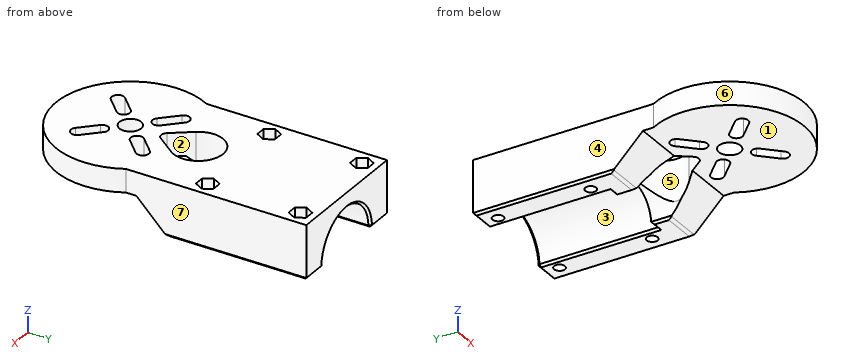
```python
from build123d import *

# Parameters (mm, degrees)
EXTRUDE006_DEPTH                     = 10
SKETCH006_AS_DRAWN_R                 = 9
EXTRUDE005_DEPTH                     = 27
EXTRUDE005_ONTO_SKETCH006_ROLL_ANGLE = 90
SKETCH_R                             = 3.5
SKETCH_R_2                           = 1.75
EXTRUDE_DEPTH                        = 30
SKETCH001_AS_DRAWN_R                 = 12.5
EXTRUDE004_DEPTH                     = 50
EXTRUDE004_ONTO_SKETCH001_ROLL_ANGLE = 90
EXTRUDE002_DEPTH                     = 60
SKETCH003_AS_DRAWN_W                 = 50
SKETCH003_AS_DRAWN_H                 = 17.5
EXTRUDE003_DEPTH                     = 98
EXTRUDE003_ONTO_SKETCH003_ROLL_ANGLE = 90
CHAMFER_SIZE                         = 0.7


with BuildPart() as extrude006:
    # Sketch008 → Extrude006 (new body)
    with BuildSketch(Plane(origin=(0, 40, 0), x_dir=(1, 0, 0), z_dir=(0, 0, 1))):
        Polygon((-17.625, -2.185417), (-14.375, -2.185417), (-12.75, -5), (-14.375, -7.814583), (-17.625, -7.814583), (-19.25, -5), align=None)
        Polygon((14.375, -2.185417), (17.625, -2.185417), (19.25, -5), (17.625, -7.814583), (14.375, -7.814583), (12.75, -5), align=None)
        Polygon((14.375, 27.814583), (17.625, 27.814583), (19.25, 25), (17.625, 22.185417), (14.375, 22.185417), (12.75, 25), align=None)
        Polygon((-17.625, 27.814583), (-14.375, 27.814583), (-12.75, 25), (-14.375, 22.185417), (-17.625, 22.185417), (-19.25, 25), align=None)
    extrude(amount=EXTRUDE006_DEPTH)


with BuildPart() as extrude006_1:
    # Extrude006 placement: moved
    add(extrude006.part.moved(Location((0, 0, 9))))


with BuildPart() as extrude005:
    # Sketch006 as drawn → Extrude005 (new)
    with BuildSketch(Plane.XY):
        Circle(SKETCH006_AS_DRAWN_R)
    extrude(amount=-EXTRUDE005_DEPTH)


with BuildPart() as extrude005_1:
    # Extrude005 onto Sketch006 roll: moved
    add(extrude005.part.rotate(Axis((0, 0, 0), (1, 0, 0)), EXTRUDE005_ONTO_SKETCH006_ROLL_ANGLE))


with BuildPart() as extrude005_2:
    # Extrude005 onto Sketch006 placement: moved
    add(extrude005_1.part.moved(Location((0, 33, 0))))


with BuildPart() as extrude005_3:
    # Extrude005 placement: moved
    add(extrude005_2.part.moved(Location((0, -18, 0))))


with BuildPart() as extrude_body:
    # Sketch → Extrude (new body)
    with BuildSketch(Plane.XY):
        Circle(SKETCH_R)
        with Locations((-16, 35)):
            Circle(SKETCH_R_2)
        with Locations((-16, 65)):
            Circle(SKETCH_R_2)
        with Locations((16, 65)):
            Circle(SKETCH_R_2)
        with Locations((16, 35)):
            Circle(SKETCH_R_2)
        with BuildLine():
            ThreePointArc((-12.020815, -9.192388), (-12.020815, -12.020815), (-9.192388, -12.020815))
            Line((-9.192388, -12.020815), (-4.242641, -7.071068))
            ThreePointArc((-4.242641, -7.071068), (-4.242641, -4.242641), (-7.071068, -4.242641))
            Line((-12.020815, -9.192388), (-7.071068, -4.242641))
        make_face()
        with BuildLine():
            ThreePointArc((7.071068, -4.242641), (4.242641, -4.242641), (4.242641, -7.071068))
            Line((4.242641, -7.071068), (9.192388, -12.020815))
            ThreePointArc((9.192388, -12.020815), (12.020815, -12.020815), (12.020815, -9.192388))
            Line((7.071068, -4.242641), (12.020815, -9.192388))
        make_face()
        with BuildLine():
            ThreePointArc((4.242641, 7.071068), (4.242641, 4.242641), (7.071068, 4.242641))
            Line((7.071068, 4.242641), (12.020815, 9.192388))
            ThreePointArc((12.020815, 9.192388), (12.020815, 12.020815), (9.192388, 12.020815))
            Line((4.242641, 7.071068), (9.192388, 12.020815))
        make_face()
        with BuildLine():
            ThreePointArc((-9.192388, 12.020815), (-12.020815, 12.020815), (-12.020815, 9.192388))
            Line((-12.020815, 9.192388), (-7.071068, 4.242641))
            ThreePointArc((-7.071068, 4.242641), (-4.242641, 4.242641), (-4.242641, 7.071068))
            Line((-9.192388, 12.020815), (-4.242641, 7.071068))
        make_face()
        with BuildLine():
            ThreePointArc((6.4, 17.2), (0, 30), (-6.4, 17.2))
            Line((-6.4, 17.2), (-1.6, 10.8))
            ThreePointArc((-1.6, 10.8), (0, 10), (1.6, 10.8))
            Line((6.4, 17.2), (1.6, 10.8))
        make_face()
        with BuildLine():
            ThreePointArc((-21, 11.61895), (0, -24), (21, 11.61895))
            Line((21, 70), (21, 11.61895))
            Line((30, 70), (21, 70))
            Line((30, -30), (30, 70))
            Line((-30, -30), (30, -30))
            Line((-30, 70), (-30, -30))
            Line((-21, 70), (-30, 70))
            Line((-21, 11.61895), (-21, 70))
        make_face()
    extrude(amount=EXTRUDE_DEPTH)


with BuildPart() as extrude004:
    # Sketch001 as drawn → Extrude004 (new)
    with BuildSketch(Plane.XY):
        Circle(SKETCH001_AS_DRAWN_R)
    extrude(amount=-EXTRUDE004_DEPTH)


with BuildPart() as extrude004_1:
    # Extrude004 onto Sketch001 roll: moved
    add(extrude004.part.rotate(Axis((0, 0, 0), (1, 0, 0)), EXTRUDE004_ONTO_SKETCH001_ROLL_ANGLE))


with BuildPart() as extrude004_2:
    # Extrude004 onto Sketch001 placement: moved
    add(extrude004_1.part.moved(Location((0, 32, 0))))


with BuildPart() as extrude004_3:
    # Extrude004 placement: moved
    add(extrude004_2.part.moved(Location((0, -1, 0))))


with BuildPart() as extrude002:
    # Sketch002 → Extrude002 (new body)
    with BuildSketch(Plane.YZ.offset(33)):
        Polygon((-30, 10), (15, 10), (25, 0), (-30, 0), align=None)
    extrude(amount=-EXTRUDE002_DEPTH)


with BuildPart() as chamfer_body:
    # Sketch003 as drawn → Extrude003 (new)
    with BuildSketch(Plane.XY):
        with Locations((0, 8.75)):
            Rectangle(SKETCH003_AS_DRAWN_W, SKETCH003_AS_DRAWN_H)
    extrude(amount=-EXTRUDE003_DEPTH)


with BuildPart() as chamfer_body_1:
    # Extrude003 onto Sketch003 roll: moved
    add(chamfer_body.part.rotate(Axis((0, 0, 0), (1, 0, 0)), EXTRUDE003_ONTO_SKETCH003_ROLL_ANGLE))


with BuildPart() as chamfer_body_2:
    # Extrude003 onto Sketch003 placement: moved
    add(chamfer_body_1.part.moved(Location((0, -28, 0))))

    # Cut: cut Extrude002
    add(extrude002.part, mode=Mode.SUBTRACT)

    # Cut001: cut Extrude004
    add(extrude004_3.part, mode=Mode.SUBTRACT)

    # Cut002: cut Extrude body
    add(extrude_body.part, mode=Mode.SUBTRACT)

    # Cut003: cut Extrude005
    add(extrude005_3.part, mode=Mode.SUBTRACT)

    # Cut004: cut Extrude006
    add(extrude006_1.part, mode=Mode.SUBTRACT)

    # Chamfer
    chamfer_edges = [chamfer_body_2.edges().sort_by_distance(p)[0] for p in [
        (-21, 47.5, 0),
        (16.75, 70, 0),
        (0, 70, 12.5),
        (-16.75, 70, 0),
        (21, 47.5, 0),
        (-15, 25, 0),
        (-9, 28, 0),
        (-12.5, 50.5, 0),
        (-10.75, 31, 0),
        (15, 25, 0),
        (9, 28, 0),
        (10.75, 31, 0),
        (12.5, 50.5, 0),
    ]]
    chamfer(chamfer_edges, length=CHAMFER_SIZE)


solid = chamfer_body_2.part
```
Read the model definition and answer for the solid it produces. Units are mm, in the model's axes. Face numbers are marked on the shaded views. A direction names the side the tool comes from. Coordinates: 2 decimals unless noted, no trailing zeros. Order: outer loops, then holes, each group sorted by start corner. A loop starts at its lowest first (then second) coordinate and runs counter-clockwise, first axis right, second up. Notation, with made-up numbers: (74.25, 42.5) - (113.25, 42.5) arc R23 cw to (113.25, 57.5) - close; hole circle Ø3 at (-22, -9.5). An arc over 180 degrees is marked (long way). Answer as a JSON object with one key per item and string values. Group by question number.
Item 1: Section A-A (x = 0) is taken. Give the vertices of the cut face in (y, z), plus the area to 3 significant figures.
Item 2: Consider probe 1 along Y at (x, z) = (0, 11); probe 2 along Y at (x, z) = (-16, 4); probe 3 along Y at (x, z) = (7, 16.5). Determine where each line is inside the solid, lowest interval first. Write a range as from..to.
Item 3: A tool of negligible diameter and unlimited length cuts with its end or side. For the marked faces 1, 2, 3 and 4, from which of +Z, -Z, +X, -X, +Y, -Y can it reach the whole face along a straight path? Write none if from no direction.
Item 4: Section B-B (y = 0) is taken. Give the vertices of the cut face in (x, z).
Item 5: The mould has two halves that part along Y. Classify the marked faces 5, 6 and 7: +Y half, -Y half, draft (parallel to the pull), parting line (faces both ways), or undercut.
Item 6: Section C-C (z = 2) is taken. State how many separate pieces and enclosed holes the cut face has, plus the area to 3 significant figures.
Item 7: Flat-ended cylindrical pins translate along their axes: P1, Ø3, axis at x = 16.5, y = 65.5, coming from the +Z side; P2, Ø6, axis at x = -12, y = -11.5, coming from the -Z side; P3, Ø10, axis at x = 3.5, z = 15, coming from the -Y side. Find the tip coordinate at first contact, or state that the pin passes through.
Results are:
{
 "1": {"outline": "(-24, 10) - (-3.5, 10) - (-3.5, 17.5) - (-24, 17.5) - close; (3.5, 10) - (10, 10) - (10, 17.5) - (3.5, 17.5) - close; (30, 9) - (31, 9) - (31, 12.5) - (69.3, 12.5) - (70, 13.2) - (70, 17.5) - (30, 17.5) - close", "area": "406 mm^2"},
 "2": {"probe 1": "y = -24..-3.5, 3.5..10, 30..31", "probe 2": "y = 21..33.25, 36.75..63.25, 66.75..70", "probe 3": "y = -22.96..-9.83, -4.17..4.17, 9.83..18.13, 25.87..70"},
 "3": {"face 1": "-Z, +X, -X, -Y", "face 2": "+Z, -Z", "face 3": "-Z, +Y", "face 4": "+Z, -Z, -X, +Y"},
 "4": {"outline": "(-24, 10) - (-3.5, 10) - (-3.5, 17.5) - (-24, 17.5) - close; (3.5, 10) - (24, 10) - (24, 17.5) - (3.5, 17.5) - close"},
 "5": {"face 5": "undercut", "face 6": "parting line", "face 7": "draft"},
 "6": {"separate pieces": "2", "enclosed holes": "4", "area": "832 mm^2"},
 "7": {"P1": "stops at z = 9", "P2": "stops at z = 10", "P3": "stops at y = -24"}
}
